Verification items for this drawing (mm, ordinates from the low corner). Round coordinates to 2 decimals unless told otherwise and drop trailing zeros. Loops run counter-clockwise (first coordinate to the right, second up) from the corner with the lowest first, then second, coordinate; pieces in that order, holes last. Notation, with made-up numbers: (40.5, 42) - (47.5, 42) arc R28 cw to (47.5, 64) - close; hole circle Ø5 at (35.25, 4). An arc over 180 degrees is marked (long way). Use a Markdown table: item, result. Add a question column.
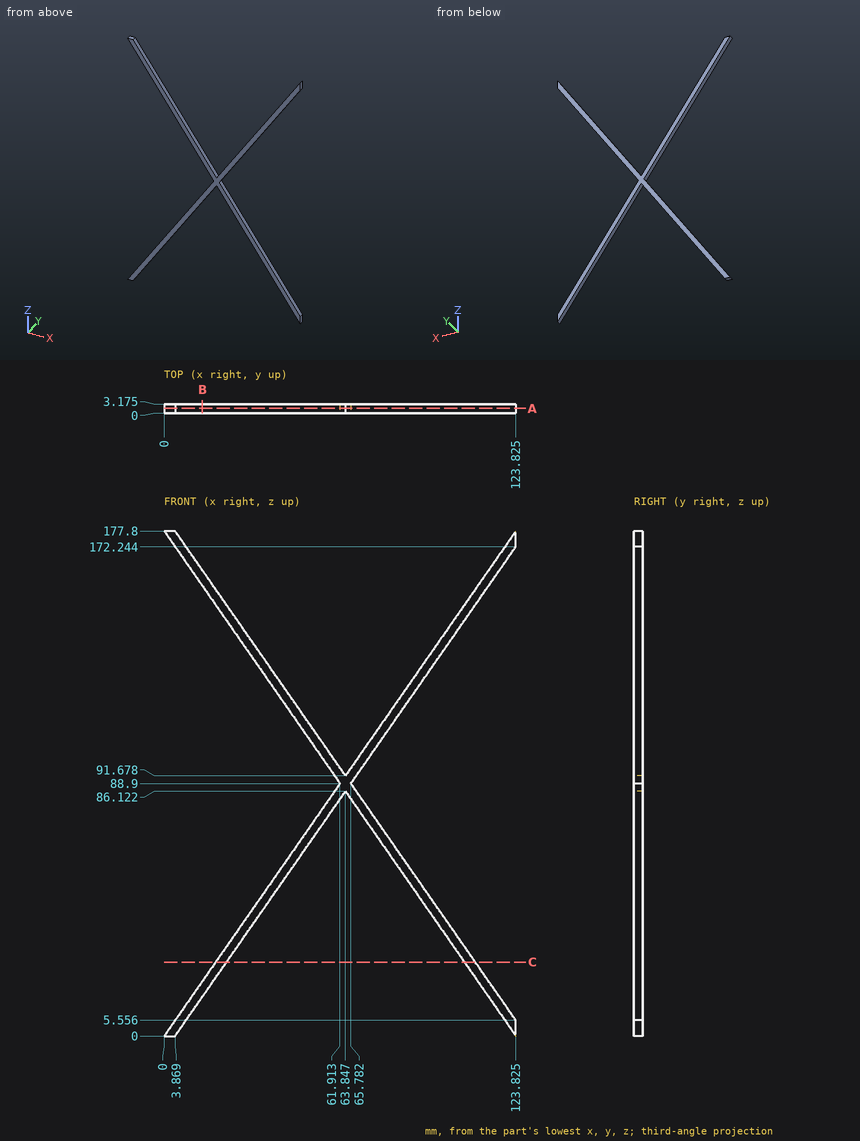
Q1. Go/stop test with flat-tipped pins: pin 1 Ø10 at (x, z) = (88, 49) entering from -Y; pin 2 Ø1 at (x, y) = (103, 1.5) entering from -Z (1 decimal); pin 3 Ø5 at (x, z) = (70.5, 108.5) entering from -Y. Record where each tip stops, or that it passes through.
Q2. Section check C-C on z = 26. Record the cut outline in (x, y) (1 decimal).
Q3. Section check A-A on y = 1.65. Record the cut outline in (x, z) (1 decimal).
Q4. Thickness scan on line 1 along X through (y, z) = (2.1, 92.5) (1 decimal); line 2 along Z through (x, y) = (115, 2.3) (1 decimal); line 3 along Z through (x, y) = (117.5, 1.95) (1 decimal). Record the ranges inside material, lowest first.
Q5. Section check B-B on x = 13.5. Record the cut outline in (y, z) (1 decimal).
Determined:
| question | item | result |
|---|---|---|
| 1 | pin 1 | stops at y = 0 |
| 1 | pin 2 | stops at z = 29.2 |
| 1 | pin 3 | passes through |
| 2 | outline | (18.1, 0) - (22, 0) - (22, 3.2) - (18.1, 3.2) - close; (105.7, 0) - (109.6, 0) - (109.6, 3.2) - (105.7, 3.2) - close |
| 3 | outline | (0, 0) - (3.9, 0) - (63.8, 86.1) - (123.8, 0) - (123.8, 5.6) - (65.8, 88.9) - (123.8, 172.2) - (123.8, 177.8) - (63.8, 91.7) - (3.9, 177.8) - (0, 177.8) - (61.9, 88.9) - close |
| 4 | line 1 | x = 59.4 to 63.3, 64.4 to 68.3 |
| 4 | line 2 | z = 12.7 to 18.2, 159.6 to 165.1 |
| 4 | line 3 | z = 9.1 to 14.6, 163.2 to 168.7 |
| 5 | outline | (0, 13.8) - (3.2, 13.8) - (3.2, 19.4) - (0, 19.4) - close; (0, 158.4) - (3.2, 158.4) - (3.2, 164) - (0, 164) - close |
